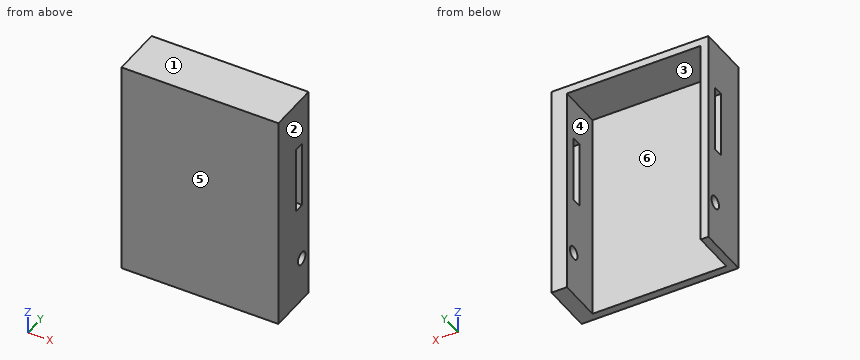
Autodesk Inventor part; units mm, degrees
ref_plane "YZ Plane" through (0, 0, 0) normal (1, 0, 0) x (0, 1, 0)
ref_plane "XZ Plane" through (0, 0, 0) normal (0, 1, 0) x (-1, 0, 0)
ref_plane "XY Plane" through (0, 0, 0) normal (0, 0, 1) x (1, 0, 0)
sketch "Sketch2" plane through (0, 0, 0) normal (0, 1, 0) x (-1, 0, 0)
  line L0 (0, 0) -> (-58, 0)
  line L1 (-58, 0) -> (-58, 85)
  line L2 (-58, 85) -> (0, 85)
  line L3 (0, 85) -> (0, 0)
  dimension "d0" = 58
  dimension "d1" = 85
extrude "Extrusion1" add sketch "Sketch2" along normal blind 20
shell "Shell1" thickness 3 removed faces 1 at (19.3333, 20, 28.3333)
sketch "Sketch4" plane through (58, 0, 0) normal (0, 0, -1) x (-1, 0, 0)
  point P0 (58, 0)
sketch "Sketch5" plane through (3, 3, 3) normal (0, 0, 1) x (1, 0, 0)
  line L0 (0, 0) -> (0, 17)
  line L1 (0, 17) -> (52, 17)
  line L2 (0, 0) -> (52, 0)
  line L3 (52, 0) -> (52, 17)
  line L4 (52, 17) -> (0, 17)
  line L5 (0, 17) -> (0, 0)
  point P0 (-3, -3)
extrude "Extrusion3" cut sketch "Sketch5" against normal blind 10
sketch "Sketch6" plane through (0, 0, 0) normal (-1, 0, 0) x (0, 0, 1)
  line L0 (40, 15.7) -> (66, 15.7)
  line L1 (66, 15.7) -> (66, 11.7)
  line L2 (66, 11.7) -> (40, 11.7)
  line L3 (40, 11.7) -> (40, 15.7)
  line L4 (0, 0) -> (0, 20)
  line L5 (0, 0) -> (85, 0)
  line L6 (85, 0) -> (85, 20)
  dimension "d19" = 26
  dimension "d20" = 4
  dimension "d22" = 11.7
  dimension "d32" = 45
sketch "Sketch7" plane through (58, 0, 85) normal (1, 0, 0) x (0, 0, -1)
  line L0 (0, 0) -> (85, 0)
  line L1 (0, 20) -> (85, 20)
  line L2 (85, 20) -> (85, 0)
  line L3 (85, 0) -> (0, 0)
  line L4 (0, 0) -> (0, 20)
extrude "Extrusion5" add sketch "Sketch7" along normal blind 3
extrude "Extrusion6" cut sketch "Sketch6" against normal through all
sketch "Sketch9" plane through (0, 0, 0) normal (-1, 0, 0) x (0, 0, 1)
  circle A0 centre (17.5212, 15.5) radius 2.5
  line L0 (0, 20) -> (85, 20)
  point P0 (0, 0)
  dimension "d33" = 5
  dimension "d36" = 2
extrude "Extrusion8" cut sketch "Sketch9" against normal through all
properties part number "breadboard box v02"
The listing builds one solid part. Answer for the finished solid, in the listing's coordinates (mm). Face numbers are marked on the shaded views. A direction names the side the tool comes from. Give positions to 0.01 mm unless a question says otherwise; leave off trailing zeros. Order: outer loops, then holes, each group sorted by start corner. A loop starts at its lowest first (then second) coordinate and runs counter-clockwise, first axis right, second up. Notation, with made-up numbers: (-11, -39.75) - (24, -39.75) arc R23 ccw to (24, -18.75) - close; hole circle Ø1 at (53.5, 37.25). An arc over 180 degrees is marked (long way). Answer in a Markdown table with one row per item. Add a question column.
Q1. Find the intervals of material crossed by line 1 along X through (y, z) = (6, 41); line 2 along Z through (x, y) = (40, 9); line 3 along Y through (x, z) = (48.5, 38), in increasing order. Write a range as [from, to].
Q2. Which of the six approach directions +Z, -Z, +X, -X, +Y, -Y give full straight-line access (tool end or side, diameter ignored) to the marked faces 5 and 6?
Q3. The part is cut by section A-A (z = 72). Determine the outline of the cut face in (x, y).
Q4. For a pull along X with two mould halves and no side action, classify the marked faces 1, 2, 3 and 4 as released by +X, released by -X, zero draft, split by the parting line, or undercut.
Q5. The part is cut by section C-C (x = 9). Determine the outline of the cut face in (y, z).
Q6. The part is cut by section B-B (y = 7.5). Determine the outline of the cut face in (x, z), then the cut area to 3 significant figures.
Q7. Given P1, Ø4.5, axis at y = 15.5, z = 17.52, coming from the -X side; P2, Ø8.5, axis at x = 32.5, y = 11, coming from the -Z side, each flat-ended and moving along its own axis, determine where each tip first touches the part or whether it passes through.
Determined:
| question | item | result |
|---|---|---|
| 1 | line 1 | x = [0, 3], [55, 61] |
| 1 | line 2 | z = [82, 85] |
| 1 | line 3 | y = [0, 3] |
| 2 | face 5 | +Z, -Z, +X, -X, -Y |
| 2 | face 6 | -Z, +Y |
| 3 | outline | (0, 0) - (61, 0) - (61, 20) - (55, 20) - (55, 3) - (3, 3) - (3, 20) - (0, 20) - close |
| 4 | face 1 | zero draft |
| 4 | face 2 | released by +X |
| 4 | face 3 | undercut |
| 4 | face 4 | undercut |
| 5 | outline | (0, 0) - (3, 0) - (3, 82) - (20, 82) - (20, 85) - (0, 85) - close |
| 6 | outline | (0, 0) - (3, 0) - (3, 82) - (55, 82) - (55, 0) - (61, 0) - (61, 85) - (0, 85) - close |
| 6 | area | 921 mm² |
| 7 | P1 | passes through |
| 7 | P2 | stops at z = 82 |
